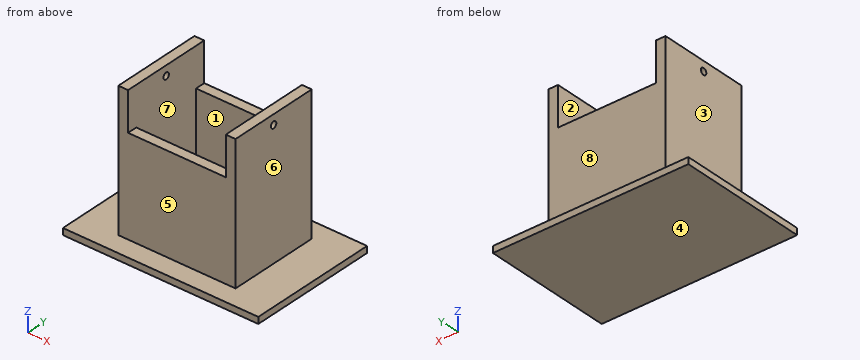
```python
from build123d import *

# Parameters (mm, degrees)
F0_W     = 30
F0_H     = 20
F1_DEPTH = 1
F2_W     = 18
F2_H     = 14
F2_W_2   = 15
F2_H_2   = 11
F3_DEPTH = 15
F4_W     = 1.5
F4_H     = 14
F5_DEPTH = 6
F6_R     = 0.5
F7_DEPTH = 24.001


with BuildPart() as f1:
    # F0 (on Top) → F1 (new body)
    with BuildSketch(Plane.XY):
        with Locations((15, 10)):
            Rectangle(F0_W, F0_H)
    extrude(amount=F1_DEPTH)

    # F2 (on face) → F3 (join)
    with BuildSketch(Plane.XY.offset(1)):
        with Locations((15, 10)):
            Rectangle(F2_W, F2_H)
        with Locations((15, 10)):
            Rectangle(F2_W_2, F2_H_2, mode=Mode.SUBTRACT)
    extrude(amount=F3_DEPTH)

    # F4 (on face) → F5 (join)
    with BuildSketch(Plane.XY.offset(16)):
        with Locations((6.75, 10)):
            Rectangle(F4_W, F4_H)
        with Locations((23.25, 10)):
            Rectangle(F4_W, F4_H)
    extrude(amount=F5_DEPTH)

    # F6 (on face) → F7 (cut, through all)
    with BuildSketch(Plane(origin=(6, 0, 0), x_dir=(0, -1, 0), z_dir=(-1, 0, 0))):
        with Locations((-10, 20.5)):
            Circle(F6_R)
    extrude(amount=-F7_DEPTH, mode=Mode.SUBTRACT)


solid = f1.part
```
Model file for the job. Use its own axes, mm. Face numbers are marked on the shaded views. A direction names the side the tool comes from. Coordinates: 2 decimals unless noted, no trailing zeros. Loops run counter-clockwise (first coordinate to the right, second up) from the corner with the lowest first, then second, coordinate; pieces in that order, holes last. Notation, with made-up numbers: (74.5, -26) - (97.5, -26) arc R14 cw to (97.5, -15) - close; hole circle Ø7 at (14, 32). An arc over 180 degrees is marked (long way). Answer as a JSON object with one key per item and string values. Group by question number.
(1) Cut at D-D (x = 5.25). Give the cut face in (y, z).
(2) Two-plate mould, pull along X, no slides. Class the marked faces 1, 2, 3 and 4: released by +X, released by -X, zero draft, split by the parting line, or undercut.
(3) Cut at C-C (y = 12.5). Give the cut face in (x, z), then the cut area to 3 significant figures.
(4) Cut at A-A (z = 13.5). Give the cut face in (x, y), then the cut area to 3 significant figures.
(5) Cut at B-B (y = 10). Give the cut face in (x, z), then the cut area to 3 significant figures.
(6) Tool access for the marked faces 5, 6, 7 and 8: list every direction of +Z, -Z, +X, -X, +Y, -Y with a clear straight run to the whole face (end or side of a thin tool).
(7) Probe line 1 along Y through (x, z) = (17, 6); line 2 along Z through (x, y) = (7.05, 10); line 3 along X through (y, z) = (15, 9.5). List the from-to ranges inside material, lowest first.
(8) Flat gauge pins, fed straight in: pin 1 (5.5 mm diameter, centred on x = 11.5, z = 14, fed in from +Y); pin 2 (12 mm diameter, centred on y = 9, z = 10.5, fed in from +X); pin 3 (2 mm diameter, centred on x = 13, y = 12, fed in from +Z). Where does each tip first touch, or does it go through?
Geometry says:
{
 "1": {"outline": "(0, 0) - (20, 0) - (20, 1) - (0, 1) - close"},
 "2": {"face 1": "undercut", "face 2": "undercut", "face 3": "released by -X", "face 4": "zero draft"},
 "3": {"outline": "(0, 0) - (30, 0) - (30, 1) - (24, 1) - (24, 22) - (22.5, 22) - (22.5, 1) - (7.5, 1) - (7.5, 22) - (6, 22) - (6, 1) - (0, 1) - close", "area": "93.0 mm^2"},
 "4": {"outline": "(6, 3) - (24, 3) - (24, 17) - (6, 17) - close; hole (7.5, 4.5) - (22.5, 4.5) - (22.5, 15.5) - (7.5, 15.5) - close", "area": "87.0 mm^2"},
 "5": {"outline": "(0, 0) - (30, 0) - (30, 1) - (24, 1) - (24, 20) - (22.5, 20) - (22.5, 1) - (7.5, 1) - (7.5, 20) - (6, 20) - (6, 1) - (0, 1) - close; (6, 21) - (7.5, 21) - (7.5, 22) - (6, 22) - close; (22.5, 21) - (24, 21) - (24, 22) - (22.5, 22) - close", "area": "90.0 mm^2"},
 "6": {"face 5": "+Z, +X, -X, -Y", "face 6": "+Z, +X, +Y, -Y", "face 7": "+Z", "face 8": "+Z, +X, -X, +Y"},
 "7": {"line 1": "y = 3 to 4.5, 15.5 to 17", "line 2": "z = 0 to 20, 21 to 22", "line 3": "x = 6 to 7.5, 22.5 to 24"},
 "8": {"pin 1": "stops at y = 17", "pin 2": "stops at x = 24", "pin 3": "stops at z = 1"}
}
